from build123d import *

# Parameters (mm, degrees)
SKETCH1_R           = 30.21838041
BOSS_EXTRUDE1_DEPTH = 38.1
BOSS_EXTRUDE2_START = 22.394673824
BOSS_EXTRUDE2_DEPTH = 22.394673824
SKETCH4_W           = 63.5
SKETCH4_H           = 76.2
BOSS_EXTRUDE4_DEPTH = 14.929782549
SKETCH5_W           = 63.5
SKETCH5_H           = 50.8
BOSS_EXTRUDE5_DEPTH = 44.789347647
SKETCH7_W           = 63.5
SKETCH7_H           = 25.4
BOSS_EXTRUDE7_DEPTH = 22.41804
SKETCH8_W           = 63.5
SKETCH8_H           = 22.42566
BOSS_EXTRUDE8_DEPTH = 22.41804


with BuildPart() as part:
    # Sketch1 → Boss-Extrude1 (new body)
    with BuildSketch(Plane.YZ):
        with Locations(Location((0, 0, 0), (0, 0, 90))):
            Circle(SKETCH1_R)
    extrude(amount=BOSS_EXTRUDE1_DEPTH)

    # Sketch2 → Boss-Extrude2 (add)
    with BuildSketch(Plane(origin=(0, 0, 0), x_dir=(0, -1, 0), z_dir=(-1, 0, 0)).offset(BOSS_EXTRUDE2_START)):
        with BuildLine():
            Line((-30.21838041, 0), (-30.21838041, 76.2))
            Line((-30.21838041, 76.2), (30.21838041, 76.2))
            Line((30.21838041, 76.2), (30.21838041, 0))
            ThreePointArc((30.21838041, 0), (0, -30.21838041), (-30.21838041, 0))
        make_face()
    extrude(amount=-BOSS_EXTRUDE2_DEPTH)

    # Sketch4 → Boss-Extrude4 (add)
    with BuildSketch(Plane.XY.offset(76.2)):
        with Locations((-11.197336912, 0)):
            Rectangle(SKETCH4_W, SKETCH4_H)
    extrude(amount=BOSS_EXTRUDE4_DEPTH)

    # Sketch5 → Boss-Extrude5 (add)
    with BuildSketch(Plane(origin=(0, 38.1, 0), x_dir=(-1, 0, 0), z_dir=(0, 1, 0))):
        with Locations((11.197336912, 101.6)):
            Rectangle(SKETCH5_W, SKETCH5_H)
    boss_extrude5 = extrude(amount=BOSS_EXTRUDE5_DEPTH)

    # Mirror1: Boss-Extrude5 across plane
    add(boss_extrude5.mirror(Plane.ZX))

    # Sketch7 → Boss-Extrude7 (add)
    with BuildSketch(Plane.XZ.offset(-38.1)):
        with Locations((-11.197336912, 114.3)):
            Rectangle(SKETCH7_W, SKETCH7_H)
    extrude(amount=BOSS_EXTRUDE7_DEPTH)

    # Sketch8 → Boss-Extrude8 (add)
    with BuildSketch(Plane(origin=(0, -38.1, 0), x_dir=(-1, 0, 0), z_dir=(0, 1, 0))):
        with Locations((11.197336912, 115.78717)):
            Rectangle(SKETCH8_W, SKETCH8_H)
    extrude(amount=BOSS_EXTRUDE8_DEPTH)


solid = part.part
For this review, take the finished solid that the model builds, in its own axes (mm). A direction names the side the tool comes from. Round coordinates to 2 decimals unless told otherwise and drop trailing zeros. Write each loop counter-clockwise with the first axis right and the second up, starting at its lowest first coordinate (ties: lowest second). Pieces come first, ordered by that corner, then holes. Notation, with made-up numbers: (89, 32.25) - (100, 32.25) arc R16 ccw to (100, 46.25) - close; hole circle Ø6 at (9.25, -21.5). An arc over 180 degrees is marked (long way). Write item = value, one per line. Start each with the question number.
1. For pin 1 Ø18 at (x, y) = (-1.5, -29) entering from -Z; pin 2 Ø4 at (x, z) = (-10.5, -0.5) entering from -Y; pin 3 Ø15 at (y, z) = (-13.5, 103.5) entering from +X, all flat-tipped, find the tip position at first contact; note any pin that passes through.
2. Consider section B-B on x = 15. State the section outline as (y, z) points.
3. Draft analysis for pull direction Z (two halves, no side actions). For faces 4 (the face through (-42.947, -1, 90)), 5 (the face through (-11, 38.1, 96)), 6 (the face through (-12, 50, 127)), state which applies: released by +Z, released by -Z, zero draft, split by the parting line, or undercut.
4. Consider section A-A on z = 112. State the section outline as (x, y) points, plus the area to 3 significant figures.
5. For faces 1 (the face through (-11, -15.682, 116)), 2 (the face through (-12, 27, 101.6)), 3 (the face through (3, 1, 76.2)), list the 3-axis set-ups (+Z, -Z, +X, -X, +Y, -Y) from which the entire face can be reached by the end or side of a thin tool; tool diameter is ignored.
6. Consider section D-D on x = -17. State the section outline as (y, z) points.
7. Wall thickness on L1, parallel to Y at x = -9, z = 99; L2, parallel to Y at x = 2, z = 116; L3, parallel to Z at x = -27.5, y = -26: over which ranges is each line inside the solid? List them lowest first.
8. Consider section C-C on y = 0. State the section outline as (x, z) points, plus the area to 3 significant figures.
Evaluation:
q1.pin_1 = -22.65
q1.pin_2 = -30.22
q1.pin_3 = 20.55
q2.outline = (-82.89, 76.2) - (82.89, 76.2) - (82.89, 127) - (15.68, 127) - (15.68, 101.6) - (38.1, 101.6) - (38.1, 91.13) - (-38.1, 91.13) - (-38.1, 104.57) - (-15.68, 104.57) - (-15.68, 127) - (-82.89, 127) - close; circle Ø60.44 at (0, 0)
q3.face_4 = zero draft
q3.face_5 = undercut
q3.face_6 = released by +Z
q4.outline = (-42.95, -82.89) - (20.55, -82.89) - (20.55, -15.68) - (-42.95, -15.68) - close; (-42.95, 15.68) - (20.55, 15.68) - (20.55, 82.89) - (-42.95, 82.89) - close
q4.area = 8,540 mm2
q5.face_1 = +Z, +X, -X
q5.face_2 = +X, -X
q5.face_3 = none
q6.outline = (-82.89, 76.2) - (-30.22, 76.2) - (-30.22, 0) arc R30.22 ccw to (30.22, 0) - (30.22, 76.2) - (82.89, 76.2) - (82.89, 127) - (15.68, 127) - (15.68, 101.6) - (38.1, 101.6) - (38.1, 91.13) - (-38.1, 91.13) - (-38.1, 104.57) - (-15.68, 104.57) - (-15.68, 127) - (-82.89, 127) - close
q7.L1 = -82.89 to -38.1, 38.1 to 82.89
q7.L2 = -82.89 to -15.68, 15.68 to 82.89
q7.L3 = 76.2 to 91.13, 104.57 to 127
q8.outline = (-42.95, 76.2) - (-22.39, 76.2) - (-22.39, -30.22) - (38.1, -30.22) - (38.1, 30.22) - (0, 30.22) - (0, 76.2) - (20.55, 76.2) - (20.55, 91.13) - (-42.95, 91.13) - close
q8.area = 5,630 mm2
